Geometry check sheet. Reference: the model listing, model coordinates, mm. A direction names the side the tool comes from. Coordinates: 2 decimals unless noted, no trailing zeros. Loops run counter-clockwise (first coordinate to the right, second up) from the corner with the lowest first, then second, coordinate; pieces in that order, holes last. Notation, with made-up numbers: (22.5, 39.5) - (32.5, 39.5) arc R34 ccw to (32.5, 76.5) - close; hole circle Ø6 at (35, -31.5). An arc over 180 degrees is marked (long way). One line per item, written item: value.
from build123d import *


with BuildPart() as part:
    # 草图3 → 旋转1 (revolve)
    with BuildSketch(Plane(origin=(0, 0, 0), x_dir=(0, 0, -1), z_dir=(1, 0, 0)), mode=Mode.PRIVATE) as revolve_1_sk:
        with BuildLine():
            Line((18.5, 0), (21.5, 0))
            Line((21.5, 0), (21.5, 4.8))
            Line((21.5, 4.8), (20.575, 5))
            Line((20.575, 5), (19.65, 5))
            Line((19.65, 5), (19.65, 4.8))
            Line((19.65, 4.8), (18.5, 4.8))
            Line((18.5, 4.8), (18.5, 5))
            Line((18.5, 5), (0, 5))
            Line((0, 5), (-18.333333333, 5))
            ThreePointArc((-18.333333333, 5), (-18.451184464, 5.048815536), (-18.5, 5.166666667))
            Line((-18.5, 5.166666667), (-18.5, 7.366666667))
            Line((-18.5, 7.366666667), (-18.633333333, 7.5))
            Line((-18.633333333, 7.5), (-21.2, 7.5))
            Line((-21.2, 7.5), (-21.5, 7.2))
            Line((-21.5, 7.2), (-21.5, 0))
            Line((-21.5, 0), (18.5, 0))
        make_face()
    revolve(revolve_1_sk.sketch.rotate(Axis((0, 0, 21.5), (0, 0, -1)), 90), axis=Axis((0, 0, 21.5), (0, 0, -1)))


solid = part.part
(1) Cross-section at A-A on x = 0. Record the cut outline in (y, z) (3 decimals), and give its area (3 significant figures).
Reply:
outline: (-7.5, 18.633) - (-7.367, 18.5) - (-5.167, 18.5) arc R0.167 cw to (-5, 18.333) - (-5, -18.5) - (-4.8, -18.5) - (-4.8, -19.65) - (-5, -19.65) - (-5, -20.575) - (-4.8, -21.5) - (4.8, -21.5) - (5, -20.575) - (5, -19.65) - (4.8, -19.65) - (4.8, -18.5) - (5, -18.5) - (5, 18.333) arc R0.167 cw to (5.167, 18.5) - (7.367, 18.5) - (7.5, 18.633) - (7.5, 21.2) - (7.2, 21.5) - (-7.2, 21.5) - (-7.5, 21.2) - close
area: 444 mm2
(2) Cross-section at C-C on z = 15.5. Record the cut outline in (x, y), and give its area (3 significant figures).
Reply:
outline: circle Ø10 at (0, 0)
area: 78.5 mm2
(3) Go/stop test with flat-tipped pins: pin 1 Ø2 at (x, z) = (5.5, -17) entering from +Y; pin 2 Ø3 at (y, z) = (-4, -17) entering from -X; pin 3 Ø6 at (x, z) = (-4, -7) entering from +Y; pin 4 Ø4 at (x, y) = (4.5, -3) entering from -Z. Record where each tip stops, or that it passes through.
Reply:
pin 1: y = 2.18
pin 2: x = -4.33
pin 3: y = 4.9
pin 4: z = -21.5
(4) Release check for a two-part mould opening along Z. For faces 1 (the face through (0, 0, 21.5)), 2 (the face through (2.58, -4.05, -19.07)), 3 (the face through (5, 2, 18.5)), 4 (the face through (-5, 0, 0)) record: pulls with the +Z half, pulls with the -Z half, needs draft (parallel to the pull), parting line crosses it, or undercut.
Reply:
face 1: pulls with the +Z half
face 2: undercut
face 3: pulls with the -Z half
face 4: needs draft
(5) Material ranges on probe 1 along Z at (x, y) = (-5.25, -4.75); probe 2 along X at (y, z) = (-0.25, -13); probe 3 along X at (y, z) = (4.25, 9), recorded low to high. Write a range as from..to.
Reply:
probe 1: 18.5..21.5
probe 2: -4.99..4.99
probe 3: -2.63..2.63
(6) Access from +Z, -Z, +X, -X, +Y, -Y to the whole of each face (thin tool, end or side, straight path). Record for faces 5 (the face through (0, 0, -21.5)), 6 (the face through (-5, 0, -20)).
Reply:
face 5: -Z, +X, -X, +Y, -Y
face 6: -Z
